Part model, mm, in its own coordinate system. A direction names the side the tool comes from. Coordinates: 2 decimals unless noted, no trailing zeros. Loops run counter-clockwise (first coordinate to the right, second up) from the corner with the lowest first, then second, coordinate; pieces in that order, holes last. Notation, with made-up numbers: M 67.25,27 L 102.25,27 A22 ccw 102.25,51 Z; hole C 76.5,14 d8. An arc over 180 degrees is marked long. Use a Markdown table: item, result. Add a question column.
1) Band-saw the part on A-A (z = -0.6). List the corners of the cut face in (x, y), plus the area to 3 significant figures.
2) Pull direction X, two halves, no side cores. Call faces 1 (the cylindrical face through (3.676, -1.718, 0.383)), 2 (the flat face through (-63.4, 1.6, 0)): released by +X, released by -X, zero draft, split by the parting line, or undercut.
3) Band-saw the part on B-B (x = -23). List the corners of the cut face in (y, z), plus the area to 3 significant figures.
4) Wall check: probe 1 along X at (y, z) = (-2, 0.15); probe 2 along X at (y, z) = (1.75, -0.1); probe 3 along X at (y, z) = (-0.75, 0.65). Give the ranges that are in metal, low to high. Write a range as from..to.
5) Pin check, flat tip, straight feed: pin 1 Ø1 at (y, z) = (-1.5, 0) entering from -X. Stop position of the tip, or through.
6) Tool access for faces 3 (the cylindrical face through (-23.241, 0.676, 0.383)), 4 (the flat face through (0, 0, 0)): list every direction of +Z, -Z, +X, -X, +Y, -Y with a clear straight run to the whole face (end or side of a thin tool).
from build123d import *

# Parameters (mm, degrees)
ESQUISSE2_R = 1


with BuildPart() as part:
    # Balayage1: sweep along a path in Esquisse1
    with BuildLine(Plane.XY) as balayage1_path:
        Line((-63.4, 1.6), (-56.371023239, -1.217761314))
        ThreePointArc((-56.371023239, -1.217761314), (-55.440643854, -1.352684575), (-54.551404356, -1.047621953))
        Line((-54.551404356, -1.047621953), (-50.891949681, 1.286251527))
        ThreePointArc((-50.891949681, 1.286251527), (-50.376649394, 1.519961335), (-49.816516844, 1.6))
        Line((-49.816516844, 1.6), (2.6, 1.6))
        ThreePointArc((2.6, 1.6), (4.014213562, 1.014213562), (4.6, -0.4))
        Line((4.6, -0.4), (4.6, -3))
        ThreePointArc((4.6, -3), (2.3, -5.3), (0, -3))
        Line((0, -3), (0, 0))
    # Esquisse2 → Balayage1 (sweep)
    with BuildSketch(Plane(origin=(0, 0, 0), x_dir=(1, 0, 0), z_dir=(0, 1, 0))):
        Circle(ESQUISSE2_R)
    sweep(path=balayage1_path.line)


solid = part.part
Entries:
| question | item | result |
|---|---|---|
| 1 | outline | M -63.7,0.86 L -56.67,-1.96 A2.8 ccw -54.12,-1.72 L -50.46,0.61 A1.2 cw -49.82,0.8 L 2.6,0.8 A1.2 cw 3.8,-0.4 L 3.8,-3 A1.5 cw 0.8,-3 L 0.8,0 L -0.8,0 L -0.8,-3 A3.1 ccw 5.4,-3 L 5.4,-0.4 A2.8 ccw 2.6,2.4 L -49.82,2.4 A2.8 ccw -51.32,1.96 L -54.98,-0.37 A1.2 cw -56.07,-0.48 L -63.1,2.34 Z |
| 1 | area | 133 mm2 |
| 2 | face 1 | undercut |
| 2 | face 2 | released by -X |
| 3 | outline | C 1.6,0 d2 |
| 3 | area | 3.14 mm2 |
| 4 | probe 1 | -57.08..-54.22, -0.99..0.99, 3.61..5.59 |
| 4 | probe 2 | -63.34..-61.1, -52.02..4.69 |
| 4 | probe 3 | -59.58..-52.67, -0.76..0.76, 3.84..5.36 |
| 5 | pin 1 | x = -59.6 |
| 6 | face 3 | none |
| 6 | face 4 | +Z, -Z |
